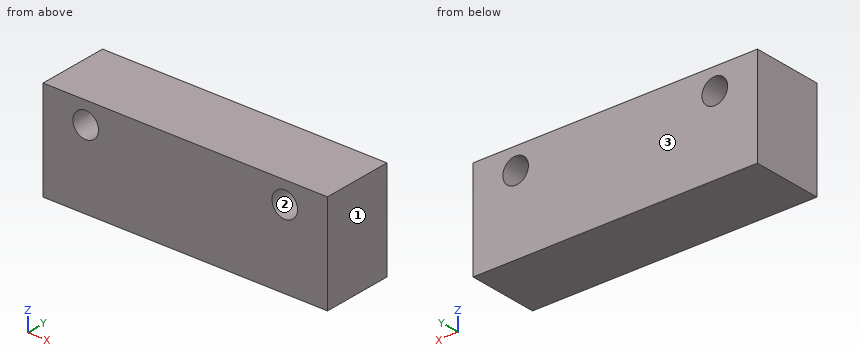
```python
from build123d import *

# Parameters (mm, degrees)
F0_W     = 100
F0_H     = 35
F0_R     = 4.5
F1_DEPTH = 25


with BuildPart() as f1:
    # F0 (on Front) → F1 (new body)
    with BuildSketch(Plane.XZ):
        Rectangle(F0_W, F0_H)
        with Locations((-35, 9.883461)):
            Circle(F0_R, mode=Mode.SUBTRACT)
        with Locations((35, 9.883461)):
            Circle(F0_R, mode=Mode.SUBTRACT)
    extrude(amount=F1_DEPTH)


solid = f1.part
```
The listing builds one solid part. Answer for the finished solid, in the listing's coordinates (mm). Face numbers are marked on the shaded views. Give positions to 0.01 mm unless a question says otherwise; leave off trailing zeros. Loops run counter-clockwise (first coordinate to the right, second up) from the corner with the lowest first, then second, coordinate; pieces in that order, holes last. Notation, with made-up numbers: M 34.25,52.5 L 72.25,52.5 A28 ccw 72.25,89.5 Z; hole C 38,33 d1. An arc over 180 degrees is marked long. One line per item, written item: value.
Q1. A cutting plane is placed at B-B on y = -6.75. Determine the outline of the cut face in (x, z).
Working result:
outline: M -50,-17.5 L 50,-17.5 L 50,17.5 L -50,17.5 Z; hole C -35,9.88 d9; hole C 35,9.88 d9
Q2. A flat-ended cylindrical pin translates along its axis: P1, Ø8, axis at x = 35, z = 9.88, coming from the -Y side. Find the tip coordinate at first contact, or state that the pin passes through.
Working result:
P1: passes through
Q3. A cutting plane is placed at A-A on x = 33. Determine the outline of the cut face in (y, z), then the cut area to 3 significant figures.
Working result:
outline: M -25,-17.5 L 0,-17.5 L 0,5.85 L -25,5.85 Z; M -25,13.91 L 0,13.91 L 0,17.5 L -25,17.5 Z
area: 673 mm^2
Q4. Determine the mould class of the marked faces 1, 2 and 3 for opening direction X: +X half, -X half, draft (parallel to the pull), parting line (faces both ways), or undercut.
Working result:
face 1: +X half
face 2: undercut
face 3: draft
Q5. Find the intervals of material crossed by line 1 (X direction, y = -1.5, z = 10); line 2 (Z direction, x = -35, y = -7.25); line 3 (X direction, y = -1.5, z = 12), in increasing order. Write a range as from..to.
Working result:
line 1: x = -50..-39.5, -30.5..30.5, 39.5..50
line 2: z = -17.5..5.38, 14.38..17.5
line 3: x = -50..-38.97, -31.03..31.03, 38.97..50
